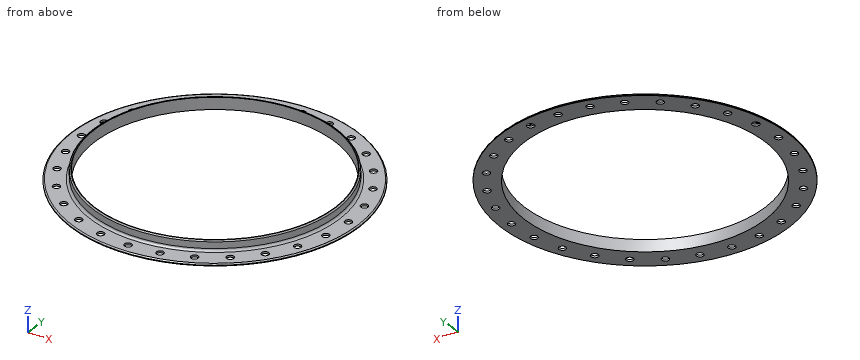
from build123d import *

# Parameters (mm, degrees)
FILLET_R           = 10
FILLET001_R        = 5
SKETCH001_R        = 15
POCKET_DEPTH       = 3473.858474
POLARPATTERN_COUNT = 28


with BuildPart() as part:
    # Sketch → Revolution (revolve)
    with BuildSketch(Plane.XZ):
        Polygon((505, 50), (505, 0), (605, 0), (605, 8), (513, 8), (513, 50), align=None)
    revolve(axis=Axis((0, 0, 0), (0, 0, 1)))

    # Fillet
    fillet_edges = [part.edges().sort_by_distance(p)[0] for p in [
        (-513, 0, 8),
    ]]
    fillet(fillet_edges, radius=FILLET_R)

    # Fillet001
    fillet001_edges = [part.edges().sort_by_distance(p)[0] for p in [
        (-605, 0, 8),
        (-513, 0, 50),
    ]]
    fillet(fillet001_edges, radius=FILLET001_R)

    # Sketch001 → Pocket (cut, through all)
    with BuildSketch(Plane.XY):
        with Locations((0, 560)):
            Circle(SKETCH001_R)
    pocket = extrude(amount=POCKET_DEPTH, mode=Mode.SUBTRACT)

    # PolarPattern: Pocket ×28 about axis
    polarpattern_axis = Axis((0, 0, 0), (0, 0, 1))
    for i in range(1, POLARPATTERN_COUNT):
        add(pocket.rotate(polarpattern_axis, i * 360 / POLARPATTERN_COUNT), mode=Mode.SUBTRACT)


solid = part.part
Read the model definition and answer for the solid it produces. Units are mm, in the model's axes. Give positions to 0.01 mm unless a question says otherwise; leave off trailing zeros. Write each loop counter-clockwise with the first axis right and the second up, starting at its lowest first coordinate (ties: lowest second). Pieces come first, ordered by that corner, then holes. Notation, with made-up numbers: (14.5, -24) - (36.5, -24) arc R27 ccw to (36.5, 6) - close; hole circle Ø1 at (83.5, -24). An arc over 180 degrees is marked (long way). Answer in a Markdown table with one row per item. Add a question column.
Item 1: Flat-ended cylindrical pins translate along their axes: P1, Ø8, axis at x = -369.5, z = 32, coming from the +Y side; P2, Ø10, axis at x = -195.5, z = 22.5, coming from the -Y side; P3, Ø18, axis at x = 124.61, y = 545.96, coming from the +Z side; P4, Ø6, axis at x = -122, z = 16.5, coming from the -Y side. Find the tip coordinate at first contact, or state that the pin passes through.
Item 2: Find the intervals of material crossed by L1, parallel to X at y = 113.5, z = 5; L2, parallel to Y at x = -305, z = 29; L3, parallel to X at y = -21, z = 37, in increasing order.
Item 3: Section A-A, the plane y = 0 is taken. Write down the section's boundary in (x, z).
Item 4: Section C-C, the plane z = 37 is taken. Write down the section's boundary in (x, y).
Recorded:
| question | item | result |
|---|---|---|
| 1 | P1 | stops at y = 359.97 |
| 1 | P2 | stops at y = -476.32 |
| 1 | P3 | passes through |
| 1 | P4 | stops at y = -499.55 |
| 2 | L1 | x = -593.83 to -556.04, -535.88 to -492.08, 492.08 to 535.88, 556.04 to 593.83 |
| 2 | L2 | y = -412.49 to -402.49, 402.49 to 412.49 |
| 2 | L3 | x = -512.57 to -504.56, 504.56 to 512.57 |
| 3 | outline | (-605, 0) - (-575, 0) - (-575, 8) - (-600, 8) arc R5 ccw to (-605, 3) - close; (-545, 0) - (-505, 0) - (-505, 50) - (-508, 50) arc R5 ccw to (-513, 45) - (-513, 18) arc R10 cw to (-523, 8) - (-545, 8) - close; (505, 0) - (545, 0) - (545, 8) - (523, 8) arc R10 cw to (513, 18) - (513, 45) arc R5 ccw to (508, 50) - (505, 50) - close; (575, 0) - (605, 0) - (605, 3) arc R5 ccw to (600, 8) - (575, 8) - close |
| 4 | outline | circle Ø1026 at (0, 0); hole circle Ø1010 at (0, 0) |
